Check sheet for the modelled part. Datum: model origin and axes. Units: mm. A direction names the side the tool comes from. Round coordinates to 2 decimals unless told otherwise and drop trailing zeros. Order: outer loops, then holes, each group sorted by start corner. A loop starts at its lowest first (then second) coordinate and runs counter-clockwise, first axis right, second up. Notation, with made-up numbers: M -11,21 L 23,21 A37 ccw 23,60 Z; hole C -32,13 d2. An arc over 180 degrees is marked long. One line per item, written item: value. Start each with the question number.
(1) Thickness scan on L1, parallel to Z at x = -15.5, y = -19; L2, parallel to Y at x = 20, z = 45; L3, parallel to Y at x = -20, z = 44.25. Record the ranges inside material, lowest first.
(2) Cross-section at D-D, the plane z = 30.5. Enter the section's corners in (x, y).
(3) Cross-section at B-B, the plane z = 9.4. Enter the section's corners in (x, y), and give its area (3 significant figures).
(4) Cross-section at A-A, the plane x = 15.5. Enter the section's corners in (y, z), and give its area (3 significant figures).
(5) Cross-section at C-C, the plane y = -20. Count the separate pieces of the cut face and the enclosed holes in it, and give its area (3 significant figures).
(6) Release check for a two-part mould opening along Z. For faces 1 (the face through (24.9, 0, 25)), 2 (the face through (-0.32, 24.3, 49.53)), 3 (the face through (19.889, 4.293, 5.075)) record: released by +Z, released by -Z, zero draft, split by the parting line, or undercut.
(7) Access from +Z, -Z, +X, -X, +Y, -Y to the whole of each face (thin tool, end or side, straight path). Record for faces 4 (the face through (19.792, -21.586, 46.044)), 5 (the face through (-19.893, 4.293, 44.725)), 6 (the face through (-14.6, -20.8, 41.6)), 7 (the face through (24.3, 0.32, 49.53)), 8 (the face through (-20.121, -22.747, 1.572)).
(8) Depth check by flat-ended pin: pin 1 Ø3 at (x, y) = (-20, -20) entering from -Z; pin 2 Ø3 at (x, y) = (-20, 20) entering from +Z; pin 3 Ø8 at (x, y) = (2.5, -4) entering from -Z. Enter the tip coordinate at first touch or a pass-through.
Autodesk Inventor part; units mm, degrees
ref_plane "YZ Plane" through (0, 0, 0) normal (1, 0, 0) x (0, 1, 0)
ref_plane "XZ Plane" through (0, 0, 0) normal (0, 1, 0) x (-1, 0, 0)
ref_plane "XY Plane" through (0, 0, 0) normal (0, 0, 1) x (1, 0, 0)
sketch "Sketch1" plane through (0, 0, 0) normal (0, 0, 1) x (1, 0, 0)
  line L0 (-24.9, 24.9) -> (24.9, 24.9)
  line L1 (24.9, 24.9) -> (24.9, -24.9)
  line L2 (24.9, -24.9) -> (-24.9, -24.9)
  line L3 (-24.9, -24.9) -> (-24.9, 24.9)
  line L4 (-24.9, 24.9) -> (24.9, -24.9) construction
  line L5 (24.9, 24.9) -> (-24.9, -24.9) construction
  line L6 (17.05, 17.05) -> (-17.05, 17.05)
  line L7 (-17.05, 17.05) -> (-17.05, -17.05)
  line L8 (-17.05, -17.05) -> (17.05, -17.05)
  line L9 (17.05, -17.05) -> (17.05, 17.05)
  point P0 (0, 0)
  dimension "d0" = 49.8
  dimension "d1" = 49.8
  dimension "d2" = 7.85
extrude "Extrusion1" add sketch "Sketch1" along normal blind 7.7 contours L0 L1 L2 L3 | L9 L8 L7 L6
sketch "Sketch2" plane through (0, 0, 7.7) normal (0, 0, 1) x (1, 0, 0)
  line L0 (24.9, 24.9) -> (-24.9, 24.9)
  line L1 (-24.9, 24.9) -> (-24.9, -24.9)
  line L2 (-24.9, -24.9) -> (24.9, -24.9)
  line L3 (24.9, -24.9) -> (24.9, 24.9)
  line L4 (17.05, -17.05) -> (24.9, -17.05)
  line L5 (24.9, -17.05) -> (24.9, -24.9)
  line L6 (24.9, -24.9) -> (17.05, -24.9)
  line L7 (17.05, -24.9) -> (17.05, -17.05)
  line L8 (17.05, 17.05) -> (-17.05, 17.05)
  line L9 (24.9, 24.9) -> (17.05, 24.9)
  line L10 (17.05, 24.9) -> (17.05, 17.05)
  line L11 (17.05, 17.05) -> (24.9, 17.05)
  line L12 (24.9, 17.05) -> (24.9, 24.9)
  line L13 (-24.9, -24.9) -> (-17.05, -24.9)
  line L14 (-17.05, -24.9) -> (-17.05, -17.05)
  line L15 (-17.05, -17.05) -> (-24.9, -17.05)
  line L16 (-24.9, -17.05) -> (-24.9, -24.9)
  line L17 (-24.9, 24.9) -> (-17.05, 24.9)
  line L18 (-17.05, 24.9) -> (-17.05, 17.05)
  line L19 (-17.05, 17.05) -> (-24.9, 17.05)
  line L20 (-24.9, 17.05) -> (-24.9, 24.9)
  point P0 (0, 0)
extrude "Extrusion2" add sketch "Sketch2" along normal blind 34.4
sketch "Sketch3" plane through (0, 0, 0) normal (0, 0, -1) x (-1, 0, 0)
  line L0 (24.9, -24.9) -> (24.9, 24.9) construction
  line L1 (24.9, 24.9) -> (-24.9, 24.9) construction
  line L2 (-24.9, -24.9) -> (24.9, -24.9) construction
  line L3 (-24.9, 24.9) -> (-24.9, -24.9) construction
  point P0 (20, 20)
  point P1 (20, -20)
  point P2 (-20, -20)
  point P3 (-20, 20)
  dimension "d_1" = 4.9
  dimension "d96" = 4.9
  dimension "d97" = 4.9
  dimension "d98" = 4.9
  dimension "d99" = 4.9
  dimension "d100" = 4.9
  dimension "d101" = 4.9
  dimension "d102" = 4.9
hole "Hole1" at (-20, 20, 0) at (-20, -20, 0) at (20, -20, 0) at (20, 20, 0) direction (0, 0, 1) diameter 2.8 end through all counterbore diameter 5.5 counterbore depth 3.1
fillet "Fillet1" radius 2 8 edges at (24.9, 24.9, 21.05) (24.9, -24.9, 21.05) (-24.9, -24.9, 21.05) (-24.9, 24.9, 21.05) (-24.9, 0, 0) (0, -24.9, 0) (24.9, 0, 0) (0, 24.9, 0)
sketch "Sketch9" plane through (0, 0, 42.1) normal (0, 0, 1) x (1, 0, 0)
  arc A0 (19.486, 18.6978) -> (18.6978, 19.486) centre (20, 20) ccw
  arc A1 (18.6978, -19.486) -> (19.486, -18.6978) centre (20, -20) ccw
  arc A2 (-19.486, -18.6978) -> (-18.6978, -19.486) centre (-20, -20) ccw
  arc A3 (-18.6978, 19.486) -> (-19.486, 18.6978) centre (-20, 20) ccw
hole "Hole2" at (20, 20, 42.1) at (-20, 20, 42.1) at (20, -20, 42.1) at (-20, -20, 42.1) direction (0, 0, -1) diameter 2.8 depth 12
sketch "Sketch15" plane through (0, 0, 0) normal (0, 0, -1) x (-1, 0, 0)
  circle A0 centre (-20, 20) radius 2.75 construction
  circle A1 centre (20, -20) radius 2.75 construction
  circle A2 centre (20, 20) radius 2.75 construction
  circle A3 centre (-20, -20) radius 2.75 construction
  line L0 (-22.9, 22.9) -> (22.9, 22.9) construction
  line L1 (-22.9, -22.9) -> (-22.9, 22.9) construction
  line L2 (22.9, -22.9) -> (-22.9, -22.9) construction
  line L3 (22.9, 22.9) -> (22.9, -22.9) construction
  line L4 (17.05, 21.1338) -> (-17.05, 21.1338) construction
  point P0 (0, 0)
  point P1 (-20.8, -14.5)
  point P2 (-14.5, -20.8)
  point P3 (14.5, -20.8)
  point P4 (20.8, -14.5)
  point P5 (20.8, 14.5)
  point P6 (14.5, 20.8)
  point P7 (-14.5, 20.8)
  point P8 (-20.8, 14.5)
hole "Hole8" [suppressed]
ref_plane "Arbeitsebene3" through (0, -17.05, 7.7) normal (1, 0, 0) x (0, 0, -1)
sketch "Skizze19" plane through (-22.9, -24.9, 42.1) normal (0, -1, 0) x (1, 0, 0)
  circle A0 centre (22.9, -17.2) radius 11.5
  circle A1 centre (38.4, -1.7) radius 1.5
  circle A2 centre (7.4, -1.7) radius 1.5
  circle A3 centre (7.4, -32.7) radius 1.5
  circle A4 centre (38.4, -32.7) radius 1.5
  point P0 (22.9, -42.1)
hole "Bohrung9" at (-15.5, -24.9, 40.4) at (15.5, -24.9, 40.4) at (15.5, -24.9, 9.4) at (-15.5, -24.9, 9.4) direction (0, 1, 0) diameter 3 end through all
sketch "Skizze20" plane through (0, 0, 42.1) normal (0, 0, 1) x (1, 0, 0)
  line L0 (24.9, 22.9) -> (24.9, -22.9)
  arc A0 (22.9, -24.9) -> (24.9, -22.9) centre (22.9, -22.9) ccw
  line L1 (22.9, -24.9) -> (-22.9, -24.9)
  arc A1 (-24.9, -22.9) -> (-22.9, -24.9) centre (-22.9, -22.9) ccw
  line L2 (-24.9, -22.9) -> (-24.9, 22.9)
  arc A2 (-22.9, 24.9) -> (-24.9, 22.9) centre (-22.9, 22.9) ccw
  line L3 (-22.9, 24.9) -> (22.9, 24.9)
  arc A3 (24.9, 22.9) -> (22.9, 24.9) centre (22.9, 22.9) ccw
  circle A4 centre (-20, 20) radius 1.6
  circle A5 centre (20, -20) radius 1.6
  circle A6 centre (20, 20) radius 1.6
  circle A7 centre (-20, -20) radius 1.6
  arc A8 (21.65, 12.3091) -> (21.65, 16.6909) centre (20.8, 14.5) ccw
  line L4 (21.65, 17.05) -> (21.65, 16.6909)
  line L5 (21.65, 17.05) -> (17.05, 17.05)
  line L6 (17.05, 17.05) -> (17.05, 21.65)
  line L7 (17.05, 21.65) -> (16.6909, 21.65)
  arc A9 (16.6909, 21.65) -> (12.3091, 21.65) centre (14.5, 20.8) ccw
  line L8 (12.3091, 21.65) -> (-12.3091, 21.65)
  arc A10 (-12.3091, 21.65) -> (-16.6909, 21.65) centre (-14.5, 20.8) ccw
  line L9 (-16.6909, 21.65) -> (-17.05, 21.65)
  line L10 (-17.05, 21.65) -> (-17.05, 17.05)
  line L11 (-17.05, 17.05) -> (-21.65, 17.05)
  line L12 (-21.65, 16.6909) -> (-21.65, 17.05)
  arc A11 (-21.65, 16.6909) -> (-21.65, 12.3091) centre (-20.8, 14.5) ccw
  line L13 (-21.65, -12.3091) -> (-21.65, 12.3091)
  arc A12 (-21.65, -12.3091) -> (-21.65, -16.6909) centre (-20.8, -14.5) ccw
  line L14 (-21.65, -17.05) -> (-21.65, -16.6909)
  line L15 (-21.65, -17.05) -> (-17.05, -17.05)
  line L16 (-17.05, -17.05) -> (-17.05, -21.65)
  line L17 (-17.05, -21.65) -> (-16.6909, -21.65)
  arc A13 (-16.6909, -21.65) -> (-12.3091, -21.65) centre (-14.5, -20.8) ccw
  line L18 (-12.3091, -21.65) -> (12.3091, -21.65)
  arc A14 (12.3091, -21.65) -> (16.6909, -21.65) centre (14.5, -20.8) ccw
  line L19 (16.6909, -21.65) -> (17.05, -21.65)
  line L20 (17.05, -21.65) -> (17.05, -17.05)
  line L21 (17.05, -17.05) -> (21.65, -17.05)
  line L22 (21.65, -16.6909) -> (21.65, -17.05)
  arc A15 (21.65, -16.6909) -> (21.65, -12.3091) centre (20.8, -14.5) ccw
  line L23 (21.65, 12.3091) -> (21.65, -12.3091)
  line L24 (-17.05, 17.05) -> (-17.05, -17.05)
  line L25 (-17.05, 17.05) -> (-17.05, -17.05)
  line L26 (-21.2838, 17.05) -> (-17.05, 17.05)
  line L27 (-17.05, 17.05) -> (17.05, 17.05)
  line L28 (17.05, 17.05) -> (17.05, -17.05)
  line L29 (17.05, -17.05) -> (-17.05, -17.05)
  line L30 (-17.05, -17.05) -> (-17.05, 17.05)
  point P0 (0, 0)
  point P1 (-17.05, -17.05)
extrude "Extrusion8" add sketch "Skizze20" along normal blind 8 contours L0 A0 L1 A1 L2 A2 L3 A3 | L23 A15 L22 L21 L28 L5 L4 A8 | L27 L10 L9 A10 L8 A9 L7 L6 | L28 L29 L24 L27 | L24 L15 L14 A12 L13 A11 L12 L11 | L20 L19 A14 L18 A13 L17 L16 L29
fillet "Rundung2" radius 2 8 edges at (-24.3142, -24.3142, 50.1) (0, -24.9, 50.1) (24.3142, -24.3142, 50.1) (24.9, 0, 50.1) (24.3142, 24.3142, 50.1) (0, 24.9, 50.1) (-24.3142, 24.3142, 50.1) (-24.9, 0, 50.1)
sketch "Skizze18" plane through (-17.05, 24.9, 7.7) normal (0, 1, 0) x (1, 0, 0)
  line L0 (-4.1, -34.35) -> (-0.1, -38.35)
  line L1 (-0.1, -38.35) -> (2.9, -38.35)
  line L2 (-4.1, -31.35) -> (2.9, -38.35)
  line L3 (-4.1, -31.35) -> (-4.1, -34.35)
  line L4 (-4.1, -34.35) -> (-0.1, -38.35)
  line L5 (38.2, -31.35) -> (38.2, -3.05)
  line L6 (38.2, -3.05) -> (31.2, 3.95)
  line L7 (31.2, 3.95) -> (2.9, 3.95)
  line L8 (2.9, 3.95) -> (-4.1, -3.05)
  line L9 (-4.1, -3.05) -> (-4.1, -31.35)
  line L10 (-4.1, -31.35) -> (2.9, -38.35)
  line L11 (2.9, -38.35) -> (31.2, -38.35)
  line L12 (31.2, -38.35) -> (38.2, -31.35)
  circle A0 centre (17.05, -17.2) radius 2.5
  circle A1 centre (1.55, -1.7) radius 1.5
  circle A2 centre (1.55, -32.7) radius 1.5
  circle A3 centre (32.55, -32.7) radius 1.5
  circle A4 centre (32.55, -1.7) radius 1.5
  circle A5 centre (17.05, -17.2) radius 4.6
  line L13 (-4.1, -31.35) -> (-4.1, -3.05)
  line L14 (2.9, -38.35) -> (-4.1, -31.35)
  line L15 (31.2, -38.35) -> (2.9, -38.35)
  line L16 (38.2, -31.35) -> (31.2, -38.35)
  line L17 (38.2, -3.05) -> (38.2, -31.35)
  line L18 (31.2, 3.95) -> (38.2, -3.05)
  line L19 (2.9, 3.95) -> (31.2, 3.95)
  line L20 (-4.1, -3.05) -> (2.9, 3.95)
  line L21 (-0.1042, 3.95) -> (34.2, 3.95)
  line L22 (38.2, -0.05) -> (38.2, -34.35)
  line L23 (34.2, -38.35) -> (-0.1042, -38.35)
  line L24 (-4.1042, -34.35) -> (-4.1042, -0.05)
  line L25 (-4.1042, -0.05) -> (-0.1042, 3.95)
  line L26 (-4.1042, -34.35) -> (-0.1042, -38.35)
  line L27 (34.2, -38.35) -> (38.2, -34.35)
  line L28 (38.2, -0.05) -> (34.2, 3.95)
  line L29 (-0.5184, 4.95) -> (-5.1042, 0.3642)
  line L30 (-5.1042, 0.3642) -> (-5.1042, -34.7642)
  line L31 (-5.1042, -34.7642) -> (-0.5184, -39.35)
  line L32 (-0.5184, -39.35) -> (34.6142, -39.35)
  line L33 (34.6142, -39.35) -> (39.2, -34.7642)
  line L34 (39.2, -34.7642) -> (39.2, 0.3642)
  line L35 (39.2, 0.3642) -> (34.6142, 4.95)
  line L36 (34.6142, 4.95) -> (-0.5184, 4.95)
  point P0 (17.05, 7.7)
  point P1 (-4.1042, 3.95)
  point P2 (38.2, -38.35)
  point P3 (38.2, 3.95)
  point P4 (-4.1042, -38.35)
  dimension "d126" = 4
  dimension "d127" = 4
  dimension "d128" = 4
  dimension "d129" = 4
  dimension "d130" = 4
  dimension "d131" = 4
  dimension "d132" = 4
  dimension "d133" = 4
  dimension "d134" = 1
extrude "Extrusion7" cut sketch "Skizze18" against normal blind 41.8 contours L3 L2 L1 L0 | L0 L23 L26 L24 L25 L21 L8 L9 L3 | L9 L8 L7 L6 L5 L12 L11 L2 | L12 L22 L27 L23 | L21 L28 L22 L6 | A0 | A1 | A2 | A3 | A4 | A5 | L36 L35 L34 L33 L32 L31 L30 L29
sketch "Skizze23" plane through (-22.9, 24.9, 2) normal (0, 1, 0) x (1, 0, 0)
  circle A0 centre (22.9, -22.9) radius 2.5
  line L0 (15.4, -1.0242) -> (30.4, -1.0242)
  line L1 (30.4, -1.0242) -> (30.4, 5.0242)
  line L2 (30.4, 5.0242) -> (15.4, 5.0242)
  line L3 (15.4, 5.0242) -> (15.4, -1.0242)
  line L4 (15.4, -1.0242) -> (30.4, 5.0242) construction
  line L5 (30.4, -1.0242) -> (15.4, 5.0242) construction
  line L6 (5.85, 2) -> (5.85, -0.75)
  line L7 (40.15, 2) -> (45.65, 2)
  line L8 (39.95, 2) -> (39.95, -0.75)
  line L9 (5.85, 2) -> (39.95, 2)
  line L10 (39.95, 2) -> (39.95, -2.8792)
  line L11 (39.95, -2.8792) -> (5.85, -2.8792)
  line L12 (5.85, -2.8792) -> (5.85, 2)
  point P0 (22.9, 2)
  point P1 (15.4, 2)
  point P2 (5.85, -0.75)
  point P3 (30.4, 2)
  dimension "d156" = 15
extrude "Extrusion10" cut sketch "Skizze23" against normal blind 42 contours L3 L9 L1 L0 | L0 L1 L9 L8 L10 L11 L12 L6 L3 | L3 L2 L1 L9
equation "\"d1\" = d0"
properties part number "55_spiralxy_slidemount_MGN9_Nema17_Body"
Values found:
1. L1: 0 to 7.9, 10.9 to 38.9, 41.9 to 50.1
1. L2: -24.9 to -21.6, -18.4 to 18.4, 21.6 to 24.9
1. L3: -24.9 to -21.6, -18.4 to -16.9
2. outline: M -24.9,-22.9 A2 ccw -22.9,-24.9 L 22.9,-24.9 A2 ccw 24.9,-22.9 L 24.9,22.9 A2 ccw 22.9,24.9 L 22.15,24.9 L 22.15,-16.9 L -22.15,-16.9 L -22.15,24.9 L -22.9,24.9 A2 ccw -24.9,22.9 Z; hole C -20,-20 d2.8; hole C 20,-20 d2.8
3. outline: M -24.9,-22.9 A2 ccw -22.9,-24.9 L -17,-24.9 L -17,-16.9 L -22.15,-16.9 L -22.15,24.9 L -22.9,24.9 A2 ccw -24.9,22.9 Z; M -14,-24.9 L 14,-24.9 L 14,-16.9 L -14,-16.9 Z; M 17,-24.9 L 22.9,-24.9 A2 ccw 24.9,-22.9 L 24.9,22.9 A2 ccw 22.9,24.9 L 22.15,24.9 L 22.15,-16.9 L 17,-16.9 Z; hole C -20,-20 d2.8; hole C 20,-20 d2.8
3. area: 564 mm^2
4. outline: M -24.9,2 A2 ccw -22.9,0 L -17.1,0 L -17.1,4.88 L -16.9,4.88 L -16.9,7.9 L -24.9,7.9 Z; M -24.9,10.9 L -16.9,10.9 L -16.9,38.9 L -24.9,38.9 Z; M -24.9,41.9 L -16.9,41.9 L -16.9,47.05 L 24.9,47.05 L 24.9,48.1 A2 ccw 22.9,50.1 L -22.9,50.1 A2 ccw -24.9,48.1 Z
4. area: 477 mm^2
5. separate pieces: 3
5. enclosed holes: 4
5. area: 2,160 mm^2
6. face 1: zero draft
6. face 2: released by +Z
6. face 3: undercut
7. face 4: +Z
7. face 5: +Y
7. face 6: +Y, -Y
7. face 7: +Z, +X, +Y, -Y
7. face 8: -Z
8. pin 1: z = 3.1
8. pin 2: z = 6.68
8. pin 3: z = 47.05
